Input: dimensioned drawing with shaded views. Units: mm. Origin: part minimum x, y, z. A direction names the side the tool comes from. Round coordinates to 2 decimals unless told otherwise and drop trailing zeros. Order: outer loops, then holes, each group sorted by start corner. A loop starts at its lowest first (then second) coordinate and runs counter-clockwise, first axis right, second up.
Item 1: Mould query, pull axis Z, two halves, no side actions, for the marked faces 3, 4 and 5. Classes: released by +Z, released by -Z, zero draft, split by the parting line, or undercut.
Item 2: Cut plane A-A on z = 16.7. Output: boundary loops of the cut face in (x, y).
Item 3: Cut plane C-C on y = 7.25. Output: boundary loops of the cut face in (x, z), then the cut area to 3 significant figures.
Item 4: Reachability of the marked faces 1 and 2 from +Z, -Z, +X, -X, +Y, -Y: full face, straight path, thin tool, end or side. Return the list, or none.
Item 5: First-contact query: pin 1 (6 mm diameter, centred on x = 13.5, z = 22.5, fed in from -Y); pin 2 (1.2 mm diameter, centred on y = 1.5, z = 10.5, fed in from +X). Flat tips, straight axial feed; report the tip coordinate or a pass-through.
Item 6: Cut plane B-B on x = 14. Output: boundary loops of the cut face in (y, z), then the cut area to 3 significant figures.
Item 7: Line query: L1, parallel to Z at x = 14, y = 10.5; L2, parallel to Y at x = 8.5, z = 13; L3, parallel to X at y = 17.75, z = 18.5. Output: solid intervals per line, ascending.
Item 8: Cut plane D-D on z = 24.5. Output: boundary loops of the cut face in (x, y), then the cut area to 3 significant figures.
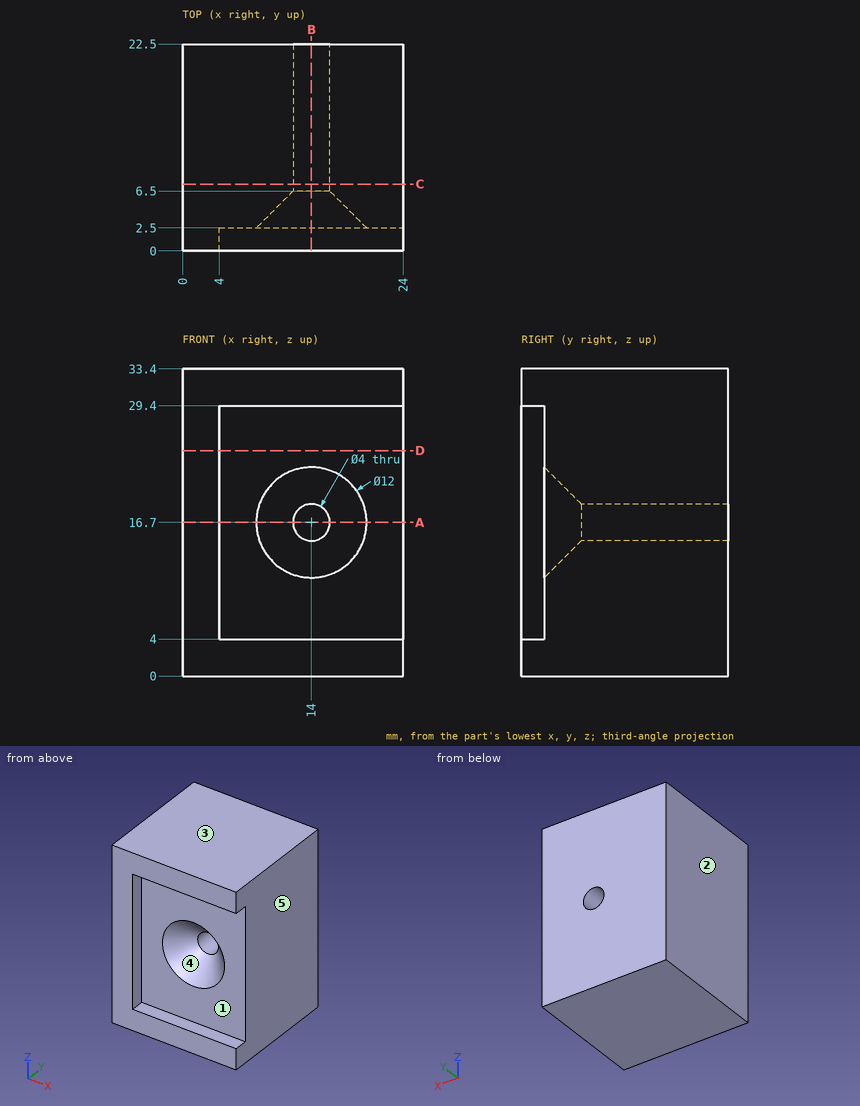
From the geometry:
1. face 3: released by +Z
1. face 4: undercut
1. face 5: zero draft
2. outline: (0, 0) - (4, 0) - (4, 2.5) - (8, 2.5) - (12, 6.5) - (12, 22.5) - (0, 22.5) - close; (16, 6.5) - (20, 2.5) - (24, 2.5) - (24, 22.5) - (16, 22.5) - close
3. outline: (0, 0) - (24, 0) - (24, 33.4) - (0, 33.4) - close; hole circle Ø4 at (14, 16.7)
3. area: 789 mm2
4. face 1: +X, -Y
4. face 2: +Z, -Z, -X, +Y, -Y
5. pin 1: stops at y = 2.5
5. pin 2: stops at x = 4
6. outline: (0, 0) - (22.5, 0) - (22.5, 14.7) - (6.5, 14.7) - (2.5, 10.7) - (2.5, 4) - (0, 4) - close; (0, 29.4) - (2.5, 29.4) - (2.5, 22.7) - (6.5, 18.7) - (22.5, 18.7) - (22.5, 33.4) - (0, 33.4) - close
6. area: 592 mm2
7. L1: z = 0 to 14.7, 18.7 to 33.4
7. L2: y = 2.5 to 22.5
7. L3: x = 0 to 13.13, 14.87 to 24
8. outline: (0, 0) - (4, 0) - (4, 2.5) - (24, 2.5) - (24, 22.5) - (0, 22.5) - close
8. area: 490 mm2
